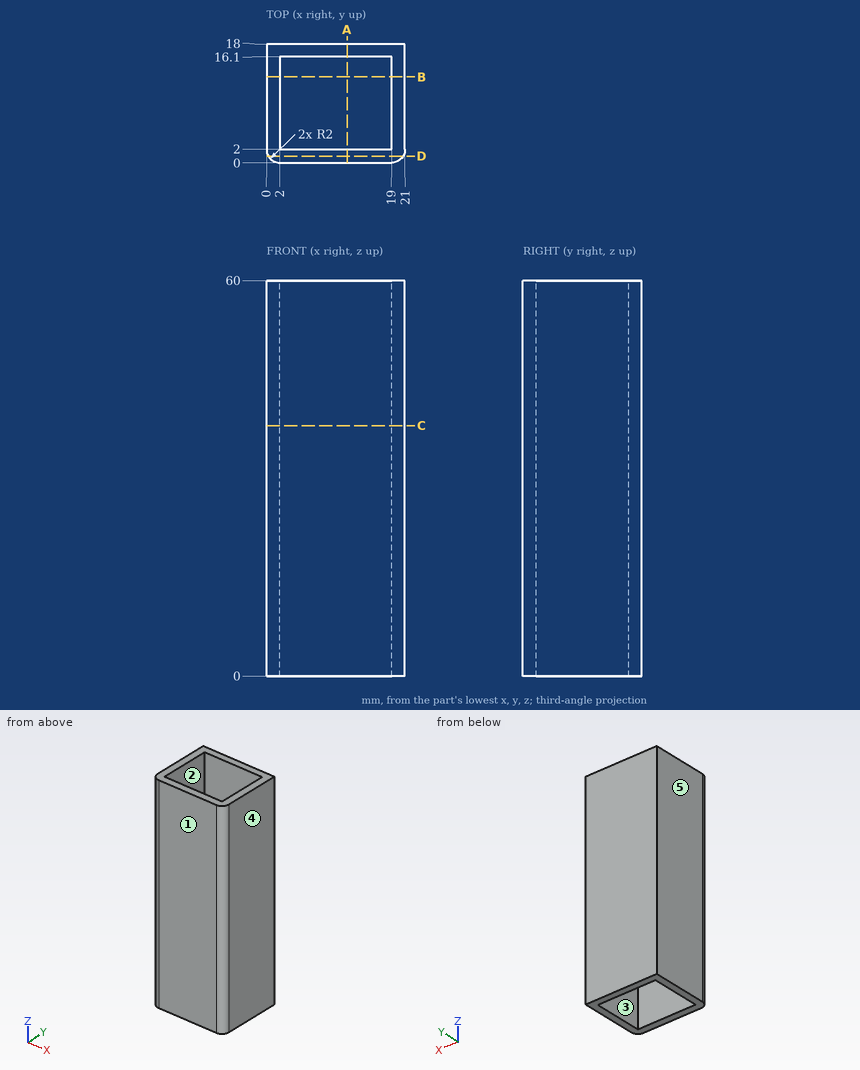
Design review of the part shown in the three views and the two pictorial views. Dimensions are in mm from the part's minimum x, y and z. A direction names the side the tool comes from. Give positions to 0.01 mm unless a question says otherwise; leave off trailing zeros. Loops run counter-clockwise (first coordinate to the right, second up) from the corner with the lowest first, then second, coordinate; pieces in that order, holes last. Notation, with made-up numbers: (-37.5, -27) -> (-29.5, -27) arc R31 cw to (-29.5, 8) -> close; hole circle Ø4 at (27, 53.5). An arc over 180 degrees is marked (long way). One line per item, written item: value.
Q1. We need section C-C on z = 38. Give the boundary of the cut face in (x, y), and give its area (3 significant figures).
Numbers:
outline: (0, 2) arc R2 ccw to (2, 0) -> (19, 0) arc R2 ccw to (21, 2) -> (21, 18) -> (0, 18) -> close; hole (2, 2) -> (19, 2) -> (19, 16.1) -> (2, 16.1) -> close
area: 137 mm^2
Q2. We need section D-D on y = 1. Give the boundary of the cut face in (x, z), and give its area (3 significant figures).
Numbers:
outline: (0.27, 0) -> (20.73, 0) -> (20.73, 60) -> (0.27, 60) -> close
area: 1,230 mm^2
Q3. We need section A-A on x = 12.25. Give the boundary of the cut face in (y, z), and give its area (3 significant figures).
Numbers:
outline: (0, 0) -> (2, 0) -> (2, 60) -> (0, 60) -> close; (16.1, 0) -> (18, 0) -> (18, 60) -> (16.1, 60) -> close
area: 234 mm^2
Q4. For pin 1 Ø8.5 at (x, z) = (12, 18.5) entering from -Y, flat-tipped, find the tip position at first contact; note if it passes through.
Numbers:
pin 1: stops at y = 0
Q5. We need section B-B on y = 13. Give the boundary of the cut face in (x, z).
Numbers:
outline: (0, 0) -> (2, 0) -> (2, 60) -> (0, 60) -> close; (19, 0) -> (21, 0) -> (21, 60) -> (19, 60) -> close
Q6. Draft analysis for pull direction X (two halves, no side actions). For the marked faces 3, 4 and 5, state which applies: pulls with the +X half, pulls with the -X half, needs draft (parallel to the pull), parting line crosses it, or undercut.
Numbers:
face 3: undercut
face 4: pulls with the +X half
face 5: pulls with the -X half
Q7. For L1, parallel to Y at x = 17, z = 51.5; L2, parallel to X at y = 4, z = 23; L3, parallel to Y at x = 1.5, z = 28, list the stretches that pass through material, from the lowest coordinate up.
Numbers:
L1: y = 0 to 2, 16.1 to 18
L2: x = 0 to 2, 19 to 21
L3: y = 0.06 to 18
Q8. Machinability: for the marked faces 1 and 2, which of the approach directions +Z, -Z, +X, -X, +Y, -Y give a long, thin tool a straight path to every point of the face, cutting with its end or side? Answer none if there is none.
Numbers:
face 1: +Z, -Z, +X, -X, -Y
face 2: +Z, -Z
